Read the model definition and answer for the solid it produces. Units are mm, in the model's axes. Face numbers are marked on the shaded views. A direction names the side the tool comes from. Give positions to 0.01 mm unless a question says otherwise; leave off trailing zeros. Write each loop counter-clockwise with the first axis right and the second up, starting at its lowest first coordinate (ties: lowest second). Pieces come first, ordered by that corner, then holes. Notation, with made-up numbers: (-4.5, 75) -> (36.5, 75) arc R12 ccw to (36.5, 92) -> close; hole circle Ø6 at (51.5, -22). An arc over 180 degrees is marked (long way). Use a Markdown table: item, result.
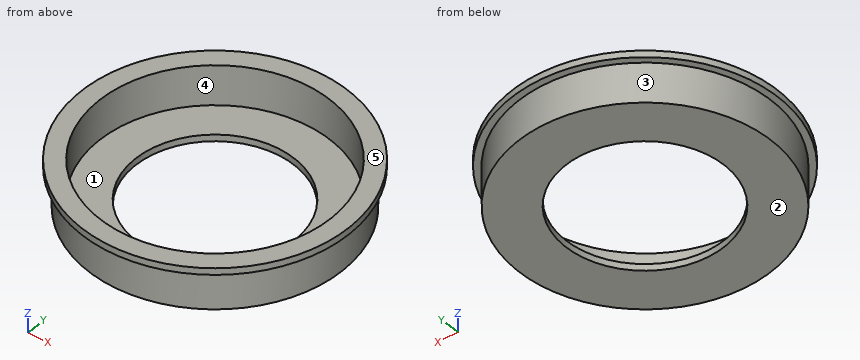
from build123d import *

# Parameters (mm, degrees)
F0_R     = 50.8
F0_R_2   = 30.226
F1_DEPTH = 2.54
F2_R     = 50.8
F2_R_2   = 43.942
F3_DEPTH = 15.24
F4_R     = 50.8
F4_R_2   = 48.26
F5_DEPTH = 15.24


with BuildPart() as f1:
    # F0 (on Top) → F1 (new body)
    with BuildSketch(Plane.XY):
        Circle(F0_R)
        Circle(F0_R_2, mode=Mode.SUBTRACT)
    extrude(amount=F1_DEPTH)

    # F2 (on face) → F3 (join)
    with BuildSketch(Plane.XY.offset(2.54)):
        Circle(F2_R)
        Circle(F2_R_2, mode=Mode.SUBTRACT)
    extrude(amount=F3_DEPTH)

    # F4 (on face) → F5 (cut)
    with BuildSketch(Plane(origin=(0, 0, 0), x_dir=(1, 0, 0), z_dir=(0, 0, -1))):
        Circle(F4_R)
        Circle(F4_R_2, mode=Mode.SUBTRACT)
    extrude(amount=-F5_DEPTH, mode=Mode.SUBTRACT)


solid = f1.part
Item 1: A cutting plane is placed at C-C (z = 8.75). Give the vertices of the cut face in (x, y).
Return value:
| item | result |
|---|---|
| outline | circle Ø96.52 at (0, 0); hole circle Ø87.88 at (0, 0) |
Item 2: A cutting plane is placed at D-D (x = 36.5). Give the vertices of the cut face in (y, z).
Return value:
| item | result |
|---|---|
| outline | (-35.33, 15.24) -> (-31.57, 15.24) -> (-31.57, 0) -> (31.57, 0) -> (31.57, 15.24) -> (35.33, 15.24) -> (35.33, 17.78) -> (24.47, 17.78) -> (24.47, 2.54) -> (-24.47, 2.54) -> (-24.47, 17.78) -> (-35.33, 17.78) -> close |
Item 3: Each of these flat-tipped pins is pushed along its axis until it touches: P1, Ø10, axis at x = 5.5, y = -36.5, coming from the +Z side; P2, Ø10, axis at x = 15, z = 13.5, coming from the +Y side; P3, Ø4, axis at x = -10, z = 2, coming from the +Y side. Where does it stop, or does it pass through?
Return value:
| item | result |
|---|---|
| P1 | z = 2.54 |
| P2 | y = 49.74 |
| P3 | y = 47.59 |
Item 4: Straight lines are drawn through the part: line 1 along Y through (x, z) = (0, 10.5); line 2 along Y through (x, z) = (0, 1.1); line 3 along Z through (x, y) = (-30.5, 24). For each, find the intervals that lie inside material, in ascending order. Write a range as [from, to].
Return value:
| item | result |
|---|---|
| line 1 | [-48.26, -43.94], [43.94, 48.26] |
| line 2 | [-48.26, -30.23], [30.23, 48.26] |
| line 3 | [0, 2.54] |
Item 5: A cutting plane is placed at A-A (y = 0). Give the vertices of the cut face in (x, z).
Return value:
| item | result |
|---|---|
| outline | (-50.8, 15.24) -> (-48.26, 15.24) -> (-48.26, 0) -> (-30.23, 0) -> (-30.23, 2.54) -> (-43.94, 2.54) -> (-43.94, 17.78) -> (-50.8, 17.78) -> close; (30.23, 0) -> (48.26, 0) -> (48.26, 15.24) -> (50.8, 15.24) -> (50.8, 17.78) -> (43.94, 17.78) -> (43.94, 2.54) -> (30.23, 2.54) -> close |
Item 6: A cutting plane is placed at B-B (x = -11.5). Give the vertices of the cut face in (y, z).
Return value:
| item | result |
|---|---|
| outline | (-49.48, 15.24) -> (-46.87, 15.24) -> (-46.87, 0) -> (-27.95, 0) -> (-27.95, 2.54) -> (-42.41, 2.54) -> (-42.41, 17.78) -> (-49.48, 17.78) -> close; (27.95, 0) -> (46.87, 0) -> (46.87, 15.24) -> (49.48, 15.24) -> (49.48, 17.78) -> (42.41, 17.78) -> (42.41, 2.54) -> (27.95, 2.54) -> close |
Item 7: A tool of negligible diameter and unlimited length cuts with its end or side. For the marked faces 4 and 5, from which of +Z, -Z, +X, -X, +Y, -Y can it reach the whole face along a straight path? Write none if from no direction.
Return value:
| item | result |
|---|---|
| face 4 | +Z |
| face 5 | +Z, +X, -X, +Y, -Y |
Item 8: For a pull along X with two mould halves and no side action, classify the marked faces 1, 2 and 3 as +X half, -X half, draft (parallel to the pull), parting line (faces both ways), or undercut.
Return value:
| item | result |
|---|---|
| face 1 | undercut |
| face 2 | draft |
| face 3 | parting line |
